```python
from build123d import *

# Parameters (mm, degrees)
SKETCH_1_W          = 76.6
SKETCH_1_H          = 36.210235533
SKETCH_1_R          = 1.6
EXTRUDE_1_DEPTH     = 3
FILLET_1_R          = 3
CUT_EXTRUDE_1_DEPTH = 102.368446486
FILLET_2_R          = 2


with BuildPart() as part:
    # 草图1 → 凸台-拉伸1 (new body)
    with BuildSketch(Plane.XY):
        with Locations((38.3, 48.219854477)):
            Rectangle(SKETCH_1_W, SKETCH_1_H)
        with Locations((9, 38.11473671)):
            Circle(SKETCH_1_R, mode=Mode.SUBTRACT)
        with Locations((9, 46.11473671)):
            Circle(SKETCH_1_R, mode=Mode.SUBTRACT)
        with Locations(Location((67.6, 38.11473671, 0), (0, 0, 180))):
            Circle(SKETCH_1_R, mode=Mode.SUBTRACT)
        with Locations(Location((67.6, 46.11473671, 0), (0, 0, 180))):
            Circle(SKETCH_1_R, mode=Mode.SUBTRACT)
    extrude(amount=EXTRUDE_1_DEPTH)

    # 圆角1
    fillet_1_edges = [part.edges().sort_by_distance(p)[0] for p in [
        (0, 66.324972243, 1.5),
        (76.6, 66.324972243, 1.5),
        (76.6, 30.11473671, 1.5),
        (0, 30.11473671, 1.5),
    ]]
    fillet(fillet_1_edges, radius=FILLET_1_R)

    # 草图2 → 切除-拉伸1 (cut, through all)
    with BuildSketch(Plane.XY.offset(3)):
        Polygon((14, 60.324972243), (35.3, 60.324972243), (14, 48.324972243), align=None)
        Polygon((62.6, 48.324972243), (41.3, 60.324972243), (62.6, 60.324972243), align=None)
        Polygon((34.3, 52.874916108), (14, 41.43829639), (14, 36.11473671), (34.3, 36.11473671), align=None)
        Polygon((62.6, 41.43829639), (62.6, 36.11473671), (42.3, 36.11473671), (42.3, 52.874916108), align=None)
    extrude(amount=-CUT_EXTRUDE_1_DEPTH, mode=Mode.SUBTRACT)

    # 圆角2
    fillet_2_edges = [part.edges().sort_by_distance(p)[0] for p in [
        (42.3, 52.874916108, 1.5),
        (62.6, 41.43829639, 1.5),
        (62.6, 36.11473671, 1.5),
        (42.3, 36.11473671, 1.5),
        (34.3, 36.11473671, 1.5),
        (14, 36.11473671, 1.5),
        (14, 41.43829639, 1.5),
        (34.3, 52.874916108, 1.5),
        (62.6, 60.324972243, 1.5),
        (62.6, 48.324972243, 1.5),
        (41.3, 60.324972243, 1.5),
        (14, 48.324972243, 1.5),
        (14, 60.324972243, 1.5),
        (35.3, 60.324972243, 1.5),
    ]]
    fillet(fillet_2_edges, radius=FILLET_2_R)


solid = part.part
```
The model under review builds one solid part; all positions refer to its coordinate system, in mm. A direction names the side the tool comes from. Round coordinates to 2 decimals unless told otherwise and drop trailing zeros. Order: outer loops, then holes, each group sorted by start corner. A loop starts at its lowest first (then second) coordinate and runs counter-clockwise, first axis right, second up. Notation, with made-up numbers: (49, 52) -> (66, 52) arc R29 cw to (66, 80) -> close; hole circle Ø9 at (58.5, 41). An arc over 180 degrees is marked (long way). Use a Markdown table: item, result.
Q1. We need section A-A on x = 67.6. Write out the cut boundary in (y, z), then the cut area to 3 significant figures.
Values:
| item | result |
|---|---|
| outline | (30.11, 0) -> (36.51, 0) -> (36.51, 3) -> (30.11, 3) -> close; (39.71, 0) -> (44.51, 0) -> (44.51, 3) -> (39.71, 3) -> close; (47.71, 0) -> (66.32, 0) -> (66.32, 3) -> (47.71, 3) -> close |
| area | 89.4 mm^2 |
Q2. We need section C-C on z = 0.7. State how many separate pieces and enclosed holes the cut face has, then the cut area to 3 significant figures.
Values:
| item | result |
|---|---|
| separate pieces | 1 |
| enclosed holes | 8 |
| area | 2,070 mm^2 |
Q3. We need section B-B on y = 52.5. Write out the cut boundary in (x, z).
Values:
| item | result |
|---|---|
| outline | (0, 0) -> (14, 0) -> (14, 3) -> (0, 3) -> close; (21.41, 0) -> (55.19, 0) -> (55.19, 3) -> (21.41, 3) -> close; (62.6, 0) -> (76.6, 0) -> (76.6, 3) -> (62.6, 3) -> close |
Q4. For line 1 (X direction, y = 38, z = 2); line 2 (Y direction, x = 9, z = 1.85); line 3 (X direction, y = 46.5, z = 2.65), list the stretches that pass through material, from the lowest coordinate up.
Values:
| item | result |
|---|---|
| line 1 | x = 0 to 7.4, 10.6 to 14, 34.3 to 42.3, 62.6 to 66, 69.2 to 76.6 |
| line 2 | y = 30.11 to 36.51, 39.71 to 44.51, 47.71 to 66.32 |
| line 3 | x = 0 to 7.45, 10.55 to 22.98, 34.3 to 42.3, 53.62 to 66.05, 69.15 to 76.6 |
Q5. Clearance check with a flat-ended pin moving along its axis: P1, Ø4, axis at x = 67.6, y = 46.11, coming from the +Z side. State where the tip first meets the part, or that it passes through.
Values:
| item | result |
|---|---|
| P1 | stops at z = 3 |
Q6. Tool access review of faces 5 (the flat face through (24, 36.115, 2)), 6 (the flat face through (38, 48, 3)): name each direction out of +Z, -Z, +X, -X, +Y, -Y from which nothing blocks a thin tool from reaching the whole face with its end or side.
Values:
| item | result |
|---|---|
| face 5 | +Z, -Z |
| face 6 | +Z, +X, -X, +Y, -Y |
Q7. Mouldability with a two-part tool opening along Y and no side actions: class faces 1 (the cylindrical face through (0.855, 31.017, 1.521)), 2 (the flat face through (38, 66.325, 1)), 3 (the cylindrical face through (8.653, 36.553, 1.479)), 4 (the flat face through (55, 60.325, 2)) as +Y half, -Y half, draft (parallel to the pull), parting line (faces both ways), or undercut.
Values:
| item | result |
|---|---|
| face 1 | -Y half |
| face 2 | +Y half |
| face 3 | undercut |
| face 4 | undercut |
